from build123d import *

# Parameters (mm, degrees)
ESQUISSE1_R      = 2
EXTRUSION1_DEPTH = 0.5
EXTRUSION2_DEPTH = 5


with BuildPart() as part:
    # Esquisse1 → Extrusion1 (new body)
    with BuildSketch(Plane(origin=(0, 0, 0), x_dir=(1, 0, 0), z_dir=(0, 1, 0))):
        with BuildLine():
            Line((-1, -10.93878444), (1, -10.93878444))
            Line((1, -10.93878444), (1, -4.582575695))
            ThreePointArc((1, -4.582575695), (1.163339973, -4.034853137), (1.6, -3.666060556))
            ThreePointArc((1.6, -3.666060556), (0, 4), (-1.6, -3.666060556))
            ThreePointArc((-1.6, -3.666060556), (-1.163339973, -4.034853137), (-1, -4.582575695))
            Line((-1, -4.582575695), (-1, -10.93878444))
        make_face()
        with Locations(Location((0, 0, 0), (0, 0, 270))):  # turned: the seam where the file's is
            Circle(ESQUISSE1_R, mode=Mode.SUBTRACT)
    extrude(amount=EXTRUSION1_DEPTH)

    # Esquisse2 → Extrusion2 (add)
    with BuildSketch(Plane.XY.offset(10.93878444)):
        with BuildLine():
            Line((1, 0), (-1, 0))
            ThreePointArc((-1, 0), (-1.599375594, 1.537610938), (0, 1.130798685))
            ThreePointArc((0, 1.130798685), (1.599375594, 1.537610938), (1, 0))
        make_face()
        with BuildLine():
            Line((-0.52344962, 0.727902261), (-0.302000478, 0.727902261))
            ThreePointArc((-0.302000478, 0.727902261), (0, 1.029902739), (0.302000478, 0.727902261))
            Line((0.302000478, 0.727902261), (0.52344962, 0.727902261))
            ThreePointArc((0.52344962, 0.727902261), (1.108344285, 1.299026833), (0.948429699, 0.497333393))
            Line((0.948429699, 0.497333393), (-0.948429699, 0.497333393))
            ThreePointArc((-0.948429699, 0.497333393), (-1.108344285, 1.299026833), (-0.52344962, 0.727902261))
        make_face(mode=Mode.SUBTRACT)
    extrude(amount=-EXTRUSION2_DEPTH)


solid = part.part
Verification items for the finished model (mm, model axes). Coordinates: 2 decimals unless noted, no trailing zeros. Order: outer loops, then holes, each group sorted by start corner. A loop starts at its lowest first (then second) coordinate and runs counter-clockwise, first axis right, second up.
1. Sectioned sample at C-C, the plane z = 8.75. Record the cut outline in (x, y), and give its area (3 significant figures).
Results found:
outline: (-1, 0) - (1, 0) arc R0.93 ccw (long way) to (0, 1.13) arc R0.93 ccw (long way) to start; hole (-0.97, 0.5) - (0.97, 0.5) arc R0.43 ccw (long way) to (0.52, 0.73) - (0.3, 0.73) arc R0.3 ccw to (-0.3, 0.73) - (-0.52, 0.73) arc R0.43 ccw (long way) to start
area: 4.14 mm2
2. Scan lines: line 1 (X direction, y = 1.1, z = 6.5); line 2 (X direction, y = 0.3, z = 0); line 3 (Y direction, x = 2.25, z = 2.5). Record each from-to range of solid material in increasing order.
Results found:
line 1: x = -1.82 to -1.29, -0.51 to 0.51, 1.29 to 1.82
line 2: x = -4 to -2, 2 to 4
line 3: y = 0 to 0.5
3. Sectioned sample at B-B, the plane y = 1.7. Record the cut outline in (x, z), and give its area (3 significant figures).
Results found:
outline: (-1.41, 5.94) - (-0.4, 5.94) - (-0.4, 10.94) - (-1.41, 10.94) - close; (0.4, 5.94) - (1.41, 5.94) - (1.41, 10.94) - (0.4, 10.94) - close
area: 10.1 mm2
4. Release check for a two-part mould opening along Y. For faces 1 (the face through (0, 0, 3)), 2 (the face through (1.09, 1.31, 8.47)), 3 (the face through (0.4, 1.3, 10.939)) record: +Y half, -Y half, draft (parallel to the pull), parting line (faces both ways), or undercut.
Results found:
face 1: -Y half
face 2: undercut
face 3: draft
5. Go/stop test with flat-tipped pins: pin 1 Ø1 at (x, z) = (2, 6.5) entering from +Y; pin 2 Ø0.6 at (y, z) = (0, 5.5) entering from +X; pin 3 Ø4 at (x, z) = (-0.5, 1) entering from +Y. Record where each tip stops, or that it passes through.
Results found:
pin 1: stops at y = 1.63
pin 2: stops at x = 1
pin 3: stops at y = 0.5
6. Sectioned sample at D-D, the plane z = 3.5. Record the cut outline in (x, y), and give its area (3 significant figures).
Results found:
outline: (-1.94, 0) - (1.94, 0) - (1.94, 0.5) - (-1.94, 0.5) - close
area: 1.94 mm2
7. Sectioned sample at A-A, the plane z = -0.25. Record the cut outline in (x, y), and give its area (3 significant figures).
Results found:
outline: (-3.99, 0) - (-1.98, 0) - (-1.98, 0.5) - (-3.99, 0.5) - close; (1.98, 0) - (3.99, 0) - (3.99, 0.5) - (1.98, 0.5) - close
area: 2.01 mm2
